from build123d import *

# Parameters (mm, degrees)
SKETCH1_W           = 16
SKETCH1_H           = 25
BOSS_EXTRUDE1_DEPTH = 1
SKETCH2_R           = 1.5
CUT_EXTRUDE1_DEPTH  = 1
SKETCH3_W           = 12.4
SKETCH3_H           = 9.9
BOSS_EXTRUDE2_DEPTH = 5
SKETCH4_R           = 1.75
BOSS_EXTRUDE3_DEPTH = 7.5


with BuildPart() as part:
    # Sketch1 → Boss-Extrude1 (new body)
    with BuildSketch(Plane.XY):
        with Locations((8, 12.5)):
            Rectangle(SKETCH1_W, SKETCH1_H)
    extrude(amount=BOSS_EXTRUDE1_DEPTH)

    # Sketch2 → Cut-Extrude1 (cut)
    with BuildSketch(Plane.XY.offset(1)):
        with Locations((2, 23)):
            Circle(SKETCH2_R)
        with Locations((14, 2)):
            Circle(SKETCH2_R)
    extrude(amount=-CUT_EXTRUDE1_DEPTH, mode=Mode.SUBTRACT)

    # Sketch3 → Boss-Extrude2 (add)
    with BuildSketch(Plane.XY.offset(1)):
        with Locations((8, 14.931642479)):
            Rectangle(SKETCH3_W, SKETCH3_H)
    extrude(amount=BOSS_EXTRUDE2_DEPTH)

    # Sketch4 → Boss-Extrude3 (add)
    with BuildSketch(Plane(origin=(0, 19.881642479, 0), x_dir=(1, 0, 0), z_dir=(0, 1, 0))):
        with Locations(Location((4.8, -3.5, 0), (0, 0, 90))):
            Circle(SKETCH4_R)
        with Locations(Location((11.2, -3.5, 0), (0, 0, 90))):
            Circle(SKETCH4_R)
    extrude(amount=BOSS_EXTRUDE3_DEPTH)


solid = part.part
Build history of the part. All positions in model axes, mm. A direction names the side the tool comes from. Round coordinates to 2 decimals unless told otherwise and drop trailing zeros. Loops run counter-clockwise (first coordinate to the right, second up) from the corner with the lowest first, then second, coordinate; pieces in that order, holes last. Notation, with made-up numbers: (36, -40) -> (44, -40) arc R18 cw to (44, -12) -> close; hole circle Ø3 at (36, 81). An arc over 180 degrees is marked (long way). One line per item, written item: value. Start each with the question number.
Q1. Cut at C-C on x = 11.2. List the corners of the cut face in (y, z), plus the area to 3 significant figures.
Q2. Cut at B-B on y = 20.5. List the corners of the cut face in (x, z).
Q3. 3-axis set-ups, long thin cutter, end or side, ignore diameter. For faces 4 (the face through (1.8, 15, 3)), 5 (the face through (7.9, 25, 0.5)), 6 (the face through (8, 19.882, 3)): which of +Z, -Z, +X, -X, +Y, -Y reach the whole face in a straight line?
Q4. Drop flat-ended pins along their axis: pin 1 Ø3 at (x, y) = (5.5, 23) entering from -Z; pin 2 Ø3 at (y, z) = (20, 3.5) entering from -X; pin 3 Ø2 at (x, y) = (14, 21.5) entering from +Z; pin 4 Ø2.5 at (x, y) = (14, 2) entering from +Z. Give the stop position or say it passes through.
Q5. Cut at D-D on x = 14.75. List the corners of the cut face in (y, z), plus the area to 3 significant figures.
Q6. Probe line 1 along Y through (x, z) = (14, 0.55); line 2 along X through (y, z) = (11.75, 3.95); line 3 along Y through (x, z) = (11, 5.6). List the from-to ranges inside material, lowest first.
Q7. Two-plate mould, pull along Z, no slides. Class faces 1 (the face through (6.51, 23.58, 3.88)), 2 (the face through (8, 9.982, 3)), 3 (the face through (8, 15, 6)): released by +Z, released by -Z, zero draft, split by the parting line, or undercut.
Q8. Cut at A-A on y = 2. List the corners of the cut face in (x, z), plus the area to 3 significant figures.
Computed:
1. outline: (0, 0) -> (25, 0) -> (25, 1) -> (19.88, 1) -> (19.88, 1.75) -> (27.38, 1.75) -> (27.38, 5.25) -> (19.88, 5.25) -> (19.88, 6) -> (9.98, 6) -> (9.98, 1) -> (0, 1) -> close
1. area: 101 mm²
2. outline: (0, 0) -> (16, 0) -> (16, 1) -> (0, 1) -> close; circle Ø3.5 at (4.8, 3.5); circle Ø3.5 at (11.2, 3.5)
3. face 4: +Z, -X, +Y, -Y
3. face 5: -Z, +X, -X, +Y
3. face 6: +Y
4. pin 1: z = 0
4. pin 2: x = 1.8
4. pin 3: z = 1
4. pin 4: through
5. outline: (0, 0) -> (0.7, 0) -> (0.7, 1) -> (0, 1) -> close; (3.3, 0) -> (25, 0) -> (25, 1) -> (3.3, 1) -> close
5. area: 22.4 mm²
6. line 1: 0 to 0.5, 3.5 to 25
6. line 2: 1.8 to 14.2
6. line 3: 9.98 to 19.88
7. face 1: undercut
7. face 2: zero draft
7. face 3: released by +Z
8. outline: (0, 0) -> (12.5, 0) -> (12.5, 1) -> (0, 1) -> close; (15.5, 0) -> (16, 0) -> (16, 1) -> (15.5, 1) -> close
8. area: 13.0 mm²
